```python
from build123d import *

# Parameters (mm, degrees)
BOSS_EXTRUDE12_DEPTH = 3
SKETCH1_16_W         = 18.27
SKETCH1_16_H         = 13.8
SKETCH1_16_W_2       = 18.57
SKETCH1_16_W_3       = 32.07
BOSS_EXTRUDE13_DEPTH = 10
SKETCH1_17_W         = 13.8
SKETCH1_17_H         = 13.8
BOSS_EXTRUDE14_DEPTH = 10
FILLET1_R            = 1


with BuildPart() as part:
    # Sketch1 → Boss-Extrude12 (new body)
    with BuildSketch(Plane(origin=(0, 0, 0), x_dir=(1, 0, 0), z_dir=(0, 1, 0))):
        with BuildLine():
            ThreePointArc((90.24192642, 0), (100, 0), (100, 9.75807358))
            Line((100, 9.75807358), (91.252103749, 18.505969831))
            ThreePointArc((91.252103749, 18.505969831), (13.301158056, 86.698841944), (81.494030169, 8.747896251))
            Line((81.494030169, 8.747896251), (90.24192642, 0))
        make_face()
    extrude(amount=BOSS_EXTRUDE12_DEPTH)

    # Sketch1_16 → Boss-Extrude13 (add)
    with BuildSketch(Plane(origin=(0, 0, 0), x_dir=(1, 0, 0), z_dir=(0, 1, 0))):
        with BuildLine():
            ThreePointArc((90.24192642, 0), (100, 0), (100, 9.75807358))
            Line((100, 9.75807358), (91.252103749, 18.505969831))
            ThreePointArc((91.252103749, 18.505969831), (13.301158056, 86.698841944), (81.494030169, 8.747896251))
            Line((81.494030169, 8.747896251), (90.24192642, 0))
        make_face()
        with BuildLine():
            Line((36.2, 56.9), (10.599619291, 56.9))
            ThreePointArc((10.599619291, 56.9), (11.37337625, 60.391532017), (12.455892606, 63.8))
            Line((12.455892606, 63.8), (43.1, 63.8))
            Line((43.1, 63.8), (43.1, 77.6))
            Line((43.1, 77.6), (21.047625313, 77.6))
            ThreePointArc((21.047625313, 77.6), (90, 50), (21.047625313, 22.4))
            Line((21.047625313, 22.4), (29.3, 22.4))
            Line((29.3, 22.4), (29.3, 36.2))
            Line((29.3, 36.2), (12.455892606, 36.2))
            ThreePointArc((12.455892606, 36.2), (11.37337625, 39.608467983), (10.599619291, 43.1))
            Line((10.599619291, 43.1), (36.2, 43.1))
            Line((36.2, 43.1), (36.2, 56.9))
        make_face(mode=Mode.SUBTRACT)
        with Locations((59.135, 70.7)):
            Rectangle(SKETCH1_16_W, SKETCH1_16_H)
        with Locations((73.085, 50)):
            Rectangle(SKETCH1_16_W_2, SKETCH1_16_H)
        with Locations((52.235, 29.3)):
            Rectangle(SKETCH1_16_W_3, SKETCH1_16_H)
    extrude(amount=BOSS_EXTRUDE13_DEPTH)

    # Sketch1_17 → Boss-Extrude14 (add)
    with BuildSketch(Plane(origin=(0, 0, 0), x_dir=(1, 0, 0), z_dir=(0, 1, 0))):
        with Locations((50, 50)):
            Rectangle(SKETCH1_17_W, SKETCH1_17_H)
    extrude(amount=BOSS_EXTRUDE14_DEPTH)

    # Fillet1
    fillet1_edges = [part.edges().sort_by_distance(p)[0] for p in [
        (43.1, 3, -50),
        (50, 3, -43.1),
        (56.9, 3, -50),
        (50, 3, -56.9),
        (50, 3, -70.7),
        (59.135, 3, -63.8),
        (68.27, 3, -70.7),
        (59.135, 3, -77.6),
        (36.2, 3, -29.3),
        (52.235, 3, -22.4),
        (68.27, 3, -29.3),
        (52.235, 3, -36.2),
        (63.8, 3, -50),
        (73.085, 3, -43.1),
        (82.37, 3, -50),
        (73.085, 3, -56.9),
        (23.399809646, 3, -43.1),
        (27.777946303, 3, -63.8),
        (25.173812657, 3, -22.4),
        (11.37337625, 3, -39.608467983),
        (36.2, 3, -50),
        (23.399809646, 3, -56.9),
        (11.37337625, 3, -60.391532017),
        (43.1, 3, -70.7),
        (32.073812657, 3, -77.6),
        (90, 3, -50),
        (29.3, 3, -29.3),
        (20.877946303, 3, -36.2),
    ]]
    fillet(fillet1_edges, radius=FILLET1_R)


solid = part.part
```
The model under review builds one solid part; all positions refer to its coordinate system, in mm. A direction names the side the tool comes from. Round coordinates to 2 decimals unless told otherwise and drop trailing zeros. Write each loop counter-clockwise with the first axis right and the second up, starting at its lowest first coordinate (ties: lowest second). Pieces come first, ordered by that corner, then holes.
(1) Machinability: for faces 4 (the flat face through (95.69, 4.93, -14.07)), 5 (the flat face through (26, 10, -51)), 6 (the flat face through (56.9, 7, -50)), which of the approach directions +Z, -Z, +X, -X, +Y, -Y give a long, thin tool a straight path to every point of the face, cutting with its end or side? Answer none if there is none.
(2) Mouldability with a two-part tool opening along Z and no side actions: class faces 1 (the flat face through (50, 10, -50)), 2 (the flat face through (85.807, 4.93, -4.435)), 3 (the flat face through (52, 7, -22.4)) as +Z half, -Z half, draft (parallel to the pull), parting line (faces both ways), or undercut.
(3) We need section A-A on y = 6. Give the number of separate pieces and of enclosed holes in the cut face, and give its area (3 significant figures).
(4) We need section D-D on z = -95.5. Give the boundary of the cut face in (x, y), and give its area (3 significant figures).
(5) Wall thickness on L1, parallel to Z at x = 49, y = 8.75; L2, parallel to Z at x = 50.5, y = 8; L3, parallel to X at y = 8.6, z = -50: over which ranges is each line inside the solid? List them lowest first.
(6) We need section B-B on z = -50. Give the boundary of the cut face in (x, y).
(7) Insertion check: pin 1 (1.8 mm diameter, centred on x = 26, y = 6.5, fed in from +Z); pin 2 (1.8 mm diameter, centred on x = 30, y = 6.5, fed in from +Z); pin 3 (1.5 mm diameter, centred on y = 8.5, z = -9.5, fed in from +X). Each pin has a flat end and moves straight along its axis. Give the tip position at first contact, or say it passes through.
(8) We need section C-C on x = 7.5. Give the boundary of the cut face in (y, z).
Findings below:
1. face 4: +X, +Y, -Y
1. face 5: +Z, -Z, +X, -X, +Y
1. face 6: +Y
2. face 1: draft
2. face 2: +Z half
2. face 3: undercut
3. separate pieces: 5
3. enclosed holes: 1
3. area: 5,730 mm2
4. outline: (25.03, 0) - (74.97, 0) - (74.97, 10) - (25.03, 10) - close
4. area: 499 mm2
5. L1: z = -101.89 to -89.99, -56.9 to -43.1, -36.2 to -22.4, -10.01 to 1.89
5. L2: z = -101.9 to -90, -77.6 to -63.8, -56.9 to -43.1, -36.2 to -22.4, -10 to 1.9
5. L3: x = -1.9 to 36.2, 43.1 to 56.9, 63.8 to 82.37, 90 to 101.9
6. outline: (-1.9, 0) - (101.9, 0) - (101.9, 10) - (90, 10) - (90, 4) arc R1 cw to (89, 3) - (83.37, 3) arc R1 cw to (82.37, 4) - (82.37, 10) - (63.8, 10) - (63.8, 4) arc R1 cw to (62.8, 3) - (57.9, 3) arc R1 cw to (56.9, 4) - (56.9, 10) - (43.1, 10) - (43.1, 4) arc R1 cw to (42.1, 3) - (37.2, 3) arc R1 cw to (36.2, 4) - (36.2, 10) - (-1.9, 10) - close
7. pin 1: stops at z = -3.52
7. pin 2: stops at z = -1.74
7. pin 3: stops at x = 100.83
8. outline: (0, -79.79) - (10, -79.79) - (10, -20.21) - (0, -20.21) - close
